```python
from build123d import *

# Parameters (mm, degrees)
F1_DEPTH = 50.8
F3_R     = 4.7625
F3_W     = 63.5
F3_H     = 101.6
F4_DEPTH = 12.7
F5_R     = 4.7625
F6_DEPTH = 9.525
F7_W     = 50.8
F7_H     = 130.0629
F8_DEPTH = 25.4


with BuildPart() as f1:
    # F0 (on Front) → F1 (new body)
    with BuildSketch(Plane.XZ):
        Polygon((1616.075, 9.525), (1616.075, 19.05), (0, 19.05), (0, 0), (781.05, 0), (781.05, 9.525), (831.85, 9.525), (831.85, 0), (1581.15, 0), (1581.15, 9.525), align=None)
    extrude(amount=F1_DEPTH)

    # F3 (on offset) → F4 (cut, symmetric)
    with BuildSketch(Plane.XY.offset(9.525)):
        with Locations((806.45, -25.4)):
            Circle(F3_R)
        with Locations((1606.55, -25.4)):
            Circle(F3_R)
        with Locations((581.025, -25.4)):
            Circle(F3_R)
        with Locations((539.75, 31.75)):
            Rectangle(F3_W, F3_H)
    extrude(amount=F4_DEPTH, both=True, mode=Mode.SUBTRACT)

    # F5 (on Right) → F6 (join)
    with BuildSketch(Plane.YZ):
        with Locations((-25.4, 9.525)):
            Circle(F5_R)
    extrude(amount=-F6_DEPTH)

    # F7 (on offset) → F8 (cut)
    with BuildSketch(Plane.XY.offset(9.525)):
        with Locations((1206.5, -27.952656)):
            Rectangle(F7_W, F7_H)
    extrude(amount=F8_DEPTH, mode=Mode.SUBTRACT)


solid = f1.part
```
CAD build for the part. Positions are in the model's coordinates, mm. A direction names the side the tool comes from. Give positions to 0.01 mm unless a question says otherwise; leave off trailing zeros. Write each loop counter-clockwise with the first axis right and the second up, starting at its lowest first coordinate (ties: lowest second). Pieces come first, ordered by that corner, then holes. Notation, with made-up numbers: M 12,-14.75 L 68,-14.75 A29 ccw 68,22.25 Z; hole C 22.5,61 d11. An arc over 180 degrees is marked long. Return JSON: item names as keys, results as strings. Group by question number.
(1) Drill centre lines: L1, parallel to X at y = -25, z = 3.5; L2, parallel to X at y = -4, z = 2.75; L3, parallel to X at y = -25.4, z = 15 (1 decimal). Where is each one in solid material? Low to high. Write a range as [from, to].
(2) Flat gauge pins, fed straight in: pin 1 Ø5 at (y, z) = (-32.5, 12.5) entering from -X; pin 2 Ø7.5 at (y, z) = (-33, 2.5) entering from +X; pin 3 Ø7.5 at (x, y) = (1606.55, -25.4) entering from -Z (3 decimals); pin 4 Ø15 at (x, y) = (1204.5, -30.5) entering from +Z (3 decimals). Where does each tip first touch, or does it go through?
(3) Band-saw the part on A-A (y = -38.5). Give the cut face in (x, z) (3 decimals), and give its area (3 significant figures).
(4) 3-axis set-ups, long thin cutter, end or side, ignore diameter. For faces 3 (the face through (1206, -25, 9.525)), 4 (the face through (1427, -25, 19.05)): which of +Z, -Z, +X, -X, +Y, -Y reach the whole face in a straight line?
(5) Mould opens along X. For faces 1 (the face through (1598, -25, 9.525)), 2 (the face through (812, -25, 9.525)) say: pulls with the +X half, pulls with the -X half, needs draft (parallel to the pull), parting line crosses it, or undercut.
Entries:
{
 "1": {"L1": "x = [0, 576.28], [585.77, 781.05], [831.85, 1581.15]", "L2": "x = [0, 508], [571.5, 781.05], [831.85, 1581.15]", "L3": "x = [0, 576.3], [585.8, 801.7], [811.2, 1181.1], [1231.9, 1601.8], [1611.3, 1616.1]"},
 "2": {"pin 1": "stops at x = 0", "pin 2": "stops at x = 1581.15", "pin 3": "passes through", "pin 4": "stops at z = 9.525"},
 "3": {"outline": "M 0,0 L 781.05,0 L 781.05,9.525 L 831.85,9.525 L 831.85,0 L 1581.15,0 L 1581.15,9.525 L 1616.075,9.525 L 1616.075,19.05 L 1231.9,19.05 L 1231.9,9.525 L 1181.1,9.525 L 1181.1,19.05 L 0,19.05 Z", "area": "29,500 mm^2"},
 "4": {"face 3": "+Z, +Y, -Y", "face 4": "+Z, +X, -X, +Y, -Y"},
 "5": {"face 1": "needs draft", "face 2": "undercut"}
}
